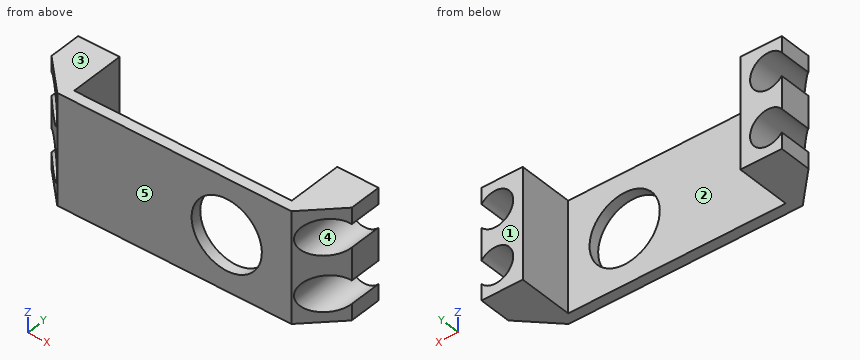
from build123d import *

# Parameters (mm, degrees)
BOSS_EXTRUDE1_DEPTH     = 20
CUT_EXTRUDE2_DEPTH      = 36.51580634
CUT_EXTRUDE2_DEPTH_BACK = 36.51580634
SKETCH2_R               = 3.25
CHAMFER1_SIZE           = 6
CUT_EXTRUDE3_DEPTH      = 36.51580634
CUT_EXTRUDE3_DEPTH_BACK = 36.51580634
SKETCH3_R               = 6.375


with BuildPart() as part:
    # Sketch1 → Boss-Extrude1 (new body)
    with BuildSketch(Plane.XY):
        Polygon((-27.25, 1), (-27.25, 10.9), (-19.75, 10.9), (-19.75, 0.9), (19.75, 0.9), (19.75, 10.9), (27.25, 10.9), (27.25, 1), (27.25, -1), (-27.25, -1), align=None)
    extrude(amount=BOSS_EXTRUDE1_DEPTH)

    # Sketch2 → Cut-Extrude2 (cut, two sides: drawn at the far end of the back side and taken through both)
    with BuildSketch(Plane(origin=(0, 0, 0), x_dir=(1, 0, 0), z_dir=(0, 1, 0)).offset(-CUT_EXTRUDE2_DEPTH_BACK)):
        with Locations((-24.75, -5)):
            Circle(SKETCH2_R)
        with Locations((24.75, -5)):
            Circle(SKETCH2_R)
        with Locations((24.75, -15)):
            Circle(SKETCH2_R)
        with Locations((-24.75, -15)):
            Circle(SKETCH2_R)
    extrude(amount=CUT_EXTRUDE2_DEPTH + CUT_EXTRUDE2_DEPTH_BACK, mode=Mode.SUBTRACT)

    # Chamfer1
    # the kernel refuses this chamfer: 6 mm, written as the material it takes off along each edge
    with BuildSketch(Plane(origin=(-27.25, -1, -15.430097928), x_dir=(-0.027495876610586206, 0.9996219169112968, 0), z_dir=(0, 0, 1))) as chamfer1_piece_1:
        Polygon((CHAMFER1_SIZE * 0.999621916911, -CHAMFER1_SIZE * 0.0274958766106), (-CHAMFER1_SIZE * 0.0274958766106, -CHAMFER1_SIZE * 0.999621916911), (0, 0), align=None)
    extrude(amount=33.78353989, mode=Mode.SUBTRACT)
    with BuildSketch(Plane(origin=(-27.25, -1, -8.353441962), x_dir=(-0.027495876610586206, 0.9996219169112968, 0), z_dir=(0, 0, 1))) as chamfer1_piece_2:
        Polygon((CHAMFER1_SIZE * 0.999621916911, -CHAMFER1_SIZE * 0.0274958766106), (-CHAMFER1_SIZE * 0.0274958766106, -CHAMFER1_SIZE * 0.999621916911), (0, 0), align=None)
    extrude(amount=36.706883924, mode=Mode.SUBTRACT)
    with BuildSketch(Plane(origin=(27.25, -1, -15.430097928), x_dir=(0.027495876610586202, 0.9996219169112968, 0), z_dir=(0, 0, 1)), Plane(origin=(27.25, -1, 1.646558038), x_dir=(0.027495876610586202, 0.9996219169112968, 0), z_dir=(0, 0, 1))) as chamfer1_piece_3:
        Polygon((CHAMFER1_SIZE * 0.999621916911, CHAMFER1_SIZE * 0.0274958766106), (-CHAMFER1_SIZE * 0.0274958766106, CHAMFER1_SIZE * 0.999621916911), (0, 0), align=None)
    extrude(amount=33.78353989, mode=Mode.SUBTRACT)
    with BuildSketch(Plane(origin=(27.25, -1, -8.353441962), x_dir=(0.027495876610586202, 0.9996219169112968, 0), z_dir=(0, 0, 1))) as chamfer1_piece_4:
        Polygon((CHAMFER1_SIZE * 0.999621916911, CHAMFER1_SIZE * 0.0274958766106), (-CHAMFER1_SIZE * 0.0274958766106, CHAMFER1_SIZE * 0.999621916911), (0, 0), align=None)
    extrude(amount=36.706883924, mode=Mode.SUBTRACT)

    # Sketch3 → Cut-Extrude3 (cut, two sides: drawn at the far end of the back side and taken through both)
    with BuildSketch(Plane(origin=(0, 0, 0), x_dir=(1, 0, 0), z_dir=(0, 1, 0)).offset(-CUT_EXTRUDE3_DEPTH_BACK)):
        with Locations(Location((9.5, -10, 0), (0, 0, 270))):
            Circle(SKETCH3_R)
    extrude(amount=CUT_EXTRUDE3_DEPTH + CUT_EXTRUDE3_DEPTH_BACK, mode=Mode.SUBTRACT)


solid = part.part
Part model, mm, in its own coordinate system. Face numbers are marked on the shaded views. A direction names the side the tool comes from. Give positions to 0.01 mm unless a question says otherwise; leave off trailing zeros. Loops run counter-clockwise (first coordinate to the right, second up) from the corner with the lowest first, then second, coordinate; pieces in that order, holes last. Notation, with made-up numbers: M 73.25,13.25 L 124.25,13.25 A13 cw 124.25,23.25 Z; hole C -21.75,20 d7. An arc over 180 degrees is marked long. Put each result on its own line as item: value. Start each with the question number.
1) Saw through at C-C (x = 24.75). List the corners of the cut face in (y, z), then the cut area to 3 significant figures.
2) Pull direction Z, two halves, no side cores. Call the marked faces 3, 4 and 5: +Z half, -Z half, draft (parallel to the pull), parting line (faces both ways), or undercut.
3) Probe probe 1 along Z at (x, y) = (-24.75, 6.75); probe 2 along X at (y, z) = (2, 5); probe 3 along Y at (x, z) = (24, 9.25). List the from-to ranges inside material, lowest first.
4) Flat gauge pin, fed straight in: pin 1 (6 mm diameter, centred on x = 2.5, z = 12.5, fed in from +Y). Where does the tip first touch, or does it go through?
5) Saw through at A-A (y = 2.5). List the corners of the cut face in (x, z), then the cut area to 3 significant figures.
6) Saw through at D-D (x = 9.5). List the corners of the cut face in (y, z) (3 decimals), then the cut area to 3 significant figures.
7) Saw through at B-B (z = 10). List the corners of the cut face in (x, y) (3 decimals), then the cut area to 3 significant figures.
8) 3-axis set-ups, long thin cutter, end or side, ignore diameter. For the marked faces 1 and 2: which of +Z, -Z, +X, -X, +Y, -Y reach the whole face in a straight line?
Numbers:
1. outline: M 2.5,0 L 10.9,0 L 10.9,1.75 L 2.5,1.75 Z; M 2.5,8.25 L 10.9,8.25 L 10.9,11.75 L 2.5,11.75 Z; M 2.5,18.25 L 10.9,18.25 L 10.9,20 L 2.5,20 Z
1. area: 58.8 mm^2
2. face 3: +Z half
2. face 4: undercut
2. face 5: draft
3. probe 1: 0 to 1.75, 8.25 to 11.75, 18.25 to 20
3. probe 2: -21.5 to -19.75, 19.75 to 21.5
3. probe 3: 1.75 to 10.9
4. pin 1: y = 0.9
5. outline: M -24.75,0 L -19.75,0 L -19.75,20 L -24.75,20 L -24.75,18.25 A3.25 cw -24.75,11.75 L -24.75,8.25 A3.25 cw -24.75,1.75 Z; M 19.75,0 L 24.75,0 L 24.75,1.75 A3.25 cw 24.75,8.25 L 24.75,11.75 A3.25 cw 24.75,18.25 L 24.75,20 L 19.75,20 Z
5. area: 134 mm^2
6. outline: M -1,0 L 0.9,0 L 0.9,3.625 L -1,3.625 Z; M -1,16.375 L 0.9,16.375 L 0.9,20 L -1,20 Z
6. area: 13.8 mm^2
7. outline: M -27.25,5 L -21.25,-1 L 3.125,-1 L 3.125,0.9 L -19.75,0.9 L -19.75,10.9 L -27.25,10.9 Z; M 15.875,-1 L 21.25,-1 L 27.25,5 L 27.25,10.9 L 19.75,10.9 L 19.75,0.9 L 15.875,0.9 Z
7. area: 193 mm^2
8. face 1: +Z, -Z, +X, -X, +Y
8. face 2: +Z, -Z, +Y
